Could you check a few things on this model? Use its own coordinates, in mm. A direction names the side the tool comes from. Coordinates: 2 decimals unless noted, no trailing zeros. Loops run counter-clockwise (first coordinate to the right, second up) from the corner with the lowest first, then second, coordinate; pieces in that order, holes last. Notation, with made-up numbers: (-7.75, 52) - (39.25, 52) arc R14 ccw to (39.25, 67) - close; hole circle Ø11 at (50, 35). An arc over 180 degrees is marked (long way). One line per item, written item: value. Start each with the question number.
(1) If we section it at A-A on x = 0: Write out the boundary of the cut face in (y, z).
(2) On a 3-axis mill with a long thin cutter (end or side, diameter ignored), from which of +Z, -Z, +X, -X, +Y, -Y can I reach the whole of each face in a straight line? I mean faces 1 (the face through (-4, 0, 3)), 2 (the face through (1.294, -1.802, 5.723)), 3 (the face through (-5.4, -1.3, -1.3)). Say none if no direction works.
(3) If we mould it in two halves opening along Z, with no side actions, what happens to faces 4 (the face through (0.9, 6.2, 0.2)), 5 (the face through (4, 0, 3)), 6 (the face through (-0.08, 0.07, 1.5)), 7 (the face through (1.7, 13, -7))? For each: pulls with the +Z half, pulls with the -Z half, needs draft (parallel to the pull), parting line crosses it, or undercut.
(4) I'm going to push flat-ended pins straight in: P1, Ø8, axis at y = -3, z = -10.5, coming from the -X side; P2, Ø5, axis at y = -6, z = 7.5, coming from the +X side; P3, Ø3, axis at x = 1, z = -3, coming from the -Y side. Where does each tip first touch, or does it pass through?
(5) If we section it at B-B on x = 3.25: Write out the boundary of the cut face in (y, z).
(6) If I drill on line 1 along Y through (x, z) = (1.5, 0); line 2 along Y through (x, z) = (1.2, 0); line 3 along X through (y, z) = (14, 8), over which ranges is the centre line in solid material (lowest first)? Write a range as from..to.
```python
from build123d import *

# Parameters (mm, degrees)
AXE_DEPTH                   = 5.4
AXE_DEPTH_BACK              = 5.4
ESQUISSE4_R                 = 3
ESQUISSE6_R                 = 4
EMPAULEMENT_ROULEMENT_DEPTH = 0.7
AXE_3MM_DEPTH               = 27.714415584
AXE_3MM_DEPTH_BACK          = 27.714415584
ESQUISSE5_R                 = 1.5
ESQUISSE7_W                 = 4.96410879
ESQUISSE7_H                 = 0.7


with BuildPart() as part:
    # Esquisse2 → Révolution1 (revolve)
    with BuildSketch(Plane.XY, mode=Mode.PRIVATE) as r_volution1_sk:
        with BuildLine():
            ThreePointArc((1.5, 18.5), (0, 17), (-1.5, 18.5))
            Line((-1.5, 18.5), (-1.7, 18.5))
            Line((-1.7, 18.5), (-1.7, 0))
            Line((-1.7, 0), (1.7, 0))
            Line((1.7, 0), (1.7, 6))
            Line((1.7, 6), (0.9, 6))
            Line((0.9, 6), (0.9, 14.4))
            Line((0.9, 14.4), (1.7, 14.4))
            Line((1.7, 14.4), (1.7, 18.5))
            Line((1.7, 18.5), (1.5, 18.5))
        make_face()
    revolve(r_volution1_sk.sketch.rotate(Axis((-1.7, 0, 0), (1, 0, 0)), 90), axis=Axis((-1.7, 0, 0), (1, 0, 0)))

    # Esquisse4 → axe (add, two sides: drawn at the far end of the back side and taken through both)
    with BuildSketch(Plane(origin=(0, 0, 0), x_dir=(0, 0, -1), z_dir=(1, 0, 0)).offset(-AXE_DEPTH_BACK)):
        Circle(ESQUISSE4_R)
    extrude(amount=AXE_DEPTH + AXE_DEPTH_BACK)

    # Esquisse6 → empaulement_roulement (add)
    with BuildSketch(Plane(origin=(1.7, 0, 0), x_dir=(0, 0, -1), z_dir=(1, 0, 0))):
        with Locations(Location((0, 0, 0), (0, 0, 180))):
            Circle(ESQUISSE6_R)
    empaulement_roulement = extrude(amount=EMPAULEMENT_ROULEMENT_DEPTH)

    # Symétrie1: empaulement_roulement across plane
    add(empaulement_roulement.mirror(Plane(origin=(0, 0, 0), x_dir=(0, 0, 1), z_dir=(1, 0, 0))))

    # Esquisse5 → axe_3mm (cut, two sides: drawn at the far end of the back side and taken through both)
    with BuildSketch(Plane(origin=(0, 0, 0), x_dir=(0, 0, -1), z_dir=(1, 0, 0)).offset(-AXE_3MM_DEPTH_BACK)):
        Circle(ESQUISSE5_R)
    extrude(amount=AXE_3MM_DEPTH + AXE_3MM_DEPTH_BACK, mode=Mode.SUBTRACT)

    # Esquisse7 → Enlèvement de matière-Révolution1 (revolve, cut)
    with BuildSketch(Plane.XY, mode=Mode.PRIVATE) as enl_vement_de_mati_re_r_volution1_sk:
        with Locations((0, 18.15)):
            Rectangle(ESQUISSE7_W, ESQUISSE7_H)
    revolve(enl_vement_de_mati_re_r_volution1_sk.sketch.rotate(Axis((0, 0, 0), (1, 0, 0)), 270), axis=Axis((0, 0, 0), (1, 0, 0)), mode=Mode.SUBTRACT)


solid = part.part
```
Values:
1. outline: circle Ø34 at (0, 0); hole circle Ø3 at (0, 0)
2. face 1: -X
2. face 2: +X
2. face 3: +Z, -Z, -X, +Y, -Y
3. face 4: undercut
3. face 5: parting line crosses it
3. face 6: undercut
3. face 7: needs draft
4. P1: stops at x = -1.7
4. P2: stops at x = 0.9
4. P3: stops at y = -17.73
5. outline: circle Ø6 at (0, 0); hole circle Ø3 at (0, 0)
6. line 1: y = -17.8..-14.4, -6..-1.5, 1.5..6, 14.4..17.8
6. line 2: y = -17.6..-14.4, -6..-1.5, 1.5..6, 14.4..17.6
6. line 3: x = -1.7..1.7
